from build123d import *

# Parameters (mm, degrees)
SKETCH3_R           = 12.7
BOSS_EXTRUDE1_DEPTH = 19.05
SHELL1_T            = -2.54
BOSS_EXTRUDE2_START = 6.35
SKETCH6_R           = 12.7
BOSS_EXTRUDE2_DEPTH = 25.4
SKETCH7_R           = 7.9375
CUT_EXTRUDE3_DEPTH  = 25.4


with BuildPart() as part:
    # Sketch2 → Revolve1 (revolve)
    with BuildSketch(Plane.XY, mode=Mode.PRIVATE) as revolve1_sk:
        with BuildLine():
            Line((0, -232.41), (49.53, -232.41))
            ThreePointArc((49.53, -232.41), (76.470768363, -221.250768363), (87.63, -194.31))
            Line((87.63, -194.31), (87.63, -156.21))
            Line((87.63, -156.21), (87.63, 156.21))
            Line((87.63, 156.21), (87.63, 194.31))
            ThreePointArc((87.63, 194.31), (76.470768363, 221.250768363), (49.53, 232.41))
            Line((49.53, 232.41), (0, 232.41))
            Line((0, 232.41), (0, -232.41))
        make_face()
    revolve(revolve1_sk.sketch.rotate(Axis((0, -232.41, 0), (0, 1, 0)), 90), axis=Axis((0, -232.41, 0), (0, 1, 0)))

    # Sketch3 → Boss-Extrude1 (add)
    with BuildSketch(Plane(origin=(0, -232.41, 0), x_dir=(-1, 0, 0), z_dir=(0, -1, 0))):
        with Locations(Location((0, 0, 0), (0, 0, 270))):
            Circle(SKETCH3_R)
    extrude(amount=BOSS_EXTRUDE1_DEPTH)

    # Shell1
    shell1_openings = [part.faces().sort_by_distance(p)[0] for p in [
        (0, -251.46, 0),
    ]]
    offset(amount=SHELL1_T, openings=shell1_openings, kind=Kind.INTERSECTION)

    # Sketch6 → Boss-Extrude2 (add)
    with BuildSketch(Plane(origin=(0, -251.46, 0), x_dir=(-1, 0, 0), z_dir=(0, -1, 0)).offset(BOSS_EXTRUDE2_START)):
        with Locations(Location((0, 0, 0), (0, 0, 270))):
            Circle(SKETCH6_R)
    extrude(amount=-BOSS_EXTRUDE2_DEPTH)

    # Sketch7 → Cut-Extrude3 (cut)
    with BuildSketch(Plane.XZ.offset(257.81)):
        with Locations(Location((0, 0, 0), (0, 0, 270))):
            Circle(SKETCH7_R)
    extrude(amount=-CUT_EXTRUDE3_DEPTH, mode=Mode.SUBTRACT)


solid = part.part
The model under review builds one solid part; all positions refer to its coordinate system, in mm. A direction names the side the tool comes from. Coordinates: 2 decimals unless noted, no trailing zeros. Write each loop counter-clockwise with the first axis right and the second up, starting at its lowest first coordinate (ties: lowest second). Pieces come first, ordered by that corner, then holes. Notation, with made-up numbers: (-27.75, -11.75) -> (-20.75, -11.75) arc R20 cw to (-20.75, 7.25) -> close; hole circle Ø6 at (71, -13). An arc over 180 degrees is marked (long way). Answer in a Markdown table with one row per item.
1. We need section B-B, the plane z = 0. State the section outline as (x, y) points.
Answers below:
| item | result |
|---|---|
| outline | (-87.63, -194.31) arc R38.1 ccw to (-49.53, -232.41) -> (-12.7, -232.41) -> (-12.7, -257.81) -> (-7.94, -257.81) -> (-7.94, -232.41) -> (-10.16, -232.41) -> (-10.16, -229.87) -> (-49.53, -229.87) arc R35.56 cw to (-85.09, -194.31) -> (-85.09, 194.31) arc R35.56 cw to (-49.53, 229.87) -> (49.53, 229.87) arc R35.56 cw to (85.09, 194.31) -> (85.09, -194.31) arc R35.56 cw to (49.53, -229.87) -> (10.16, -229.87) -> (10.16, -232.41) -> (7.94, -232.41) -> (7.94, -257.81) -> (12.7, -257.81) -> (12.7, -232.41) -> (49.53, -232.41) arc R38.1 ccw to (87.63, -194.31) -> (87.63, 194.31) arc R38.1 ccw to (49.53, 232.41) -> (-49.53, 232.41) arc R38.1 ccw to (-87.63, 194.31) -> close |
2. Clearance check with flat-ended pins moving along their axes: pin 1 Ø8 at (x, y) = (-52, 116) entering from -Z; pin 2 Ø1 at (x, z) = (47.5, 60.5) entering from -Y; pin 3 Ø5 at (x, z) = (-19, -11) entering from -Y; pin 4 Ø12 at (x, z) = (20, 46.5) entering from +Y. State where each tip first meets the part, or that it passes through.
Answers below:
| item | result |
|---|---|
| pin 1 | stops at z = -73.31 |
| pin 2 | stops at y = -221.3 |
| pin 3 | stops at y = -232.41 |
| pin 4 | stops at y = 232.41 |
3. For faces 4 (the flat face through (-1, 232.41, 1)), 5 (the flat face through (10, -232.41, 10)), 6 (the cylindrical face through (-10.074, -231.122, -1.323)), list the 3-axis set-ups (+Z, -Z, +X, -X, +Y, -Y) from which the entire face can be reached by the end or side of a thin tool; tool diameter is ignored.
Answers below:
| item | result |
|---|---|
| face 4 | +Z, -Z, +X, -X, +Y |
| face 5 | -Y |
| face 6 | none |
4. We need section A-A, the plane x = 0. State the section outline as (y, z) points, and give its area (3 significant figures).
Answers below:
| item | result |
|---|---|
| outline | (-257.81, -12.7) -> (-232.41, -12.7) -> (-232.41, -49.53) arc R38.1 ccw to (-194.31, -87.63) -> (194.31, -87.63) arc R38.1 ccw to (232.41, -49.53) -> (232.41, 49.53) arc R38.1 ccw to (194.31, 87.63) -> (-194.31, 87.63) arc R38.1 ccw to (-232.41, 49.53) -> (-232.41, 12.7) -> (-257.81, 12.7) -> (-257.81, 7.94) -> (-232.41, 7.94) -> (-232.41, 10.16) -> (-229.87, 10.16) -> (-229.87, 49.53) arc R35.56 cw to (-194.31, 85.09) -> (194.31, 85.09) arc R35.56 cw to (229.87, 49.53) -> (229.87, -49.53) arc R35.56 cw to (194.31, -85.09) -> (-194.31, -85.09) arc R35.56 cw to (-229.87, -49.53) -> (-229.87, -10.16) -> (-232.41, -10.16) -> (-232.41, -7.94) -> (-257.81, -7.94) -> close |
| area | 3,260 mm^2 |
5. Wall thickness on probe 1 along Y at (x, z) = (13, 43.5); probe 2 along X at (y, z) = (28, -3.5); probe 3 along X at (y, z) = (-241, 0): over which ranges is each line inside the solid? List them lowest first. Write a range as [from, to].
Answers below:
| item | result |
|---|---|
| probe 1 | y = [-232.41, -229.87], [229.87, 232.41] |
| probe 2 | x = [-87.56, -85.02], [85.02, 87.56] |
| probe 3 | x = [-12.7, -7.94], [7.94, 12.7] |
6. Draft analysis for pull direction Y (two halves, no side actions). For faces 1 (the cylindrical face through (85.546, 2.72, 18.996)), 2 (the flat face through (8.3, -257.81, -0.2)), 3 (the cylindrical face through (75.49, 2.72, -39.26)), state which applies: +Y half, -Y half, draft (parallel to the pull), parting line (faces both ways), or undercut.
Answers below:
| item | result |
|---|---|
| face 1 | draft |
| face 2 | -Y half |
| face 3 | undercut |
7. We need section C-C, the plane y = -218. State the section outline as (x, z) points, and give its area (3 significant figures).
Answers below:
| item | result |
|---|---|
| outline | circle Ø158.74 at (0, 0); hole circle Ø152.1 at (0, 0) |
| area | 1,620 mm^2 |
8. We need section D-D, the plane y = -153. State the section outline as (x, z) points, and give its area (3 significant figures).
Answers below:
| item | result |
|---|---|
| outline | circle Ø175.26 at (0, 0); hole circle Ø170.18 at (0, 0) |
| area | 1,380 mm^2 |
